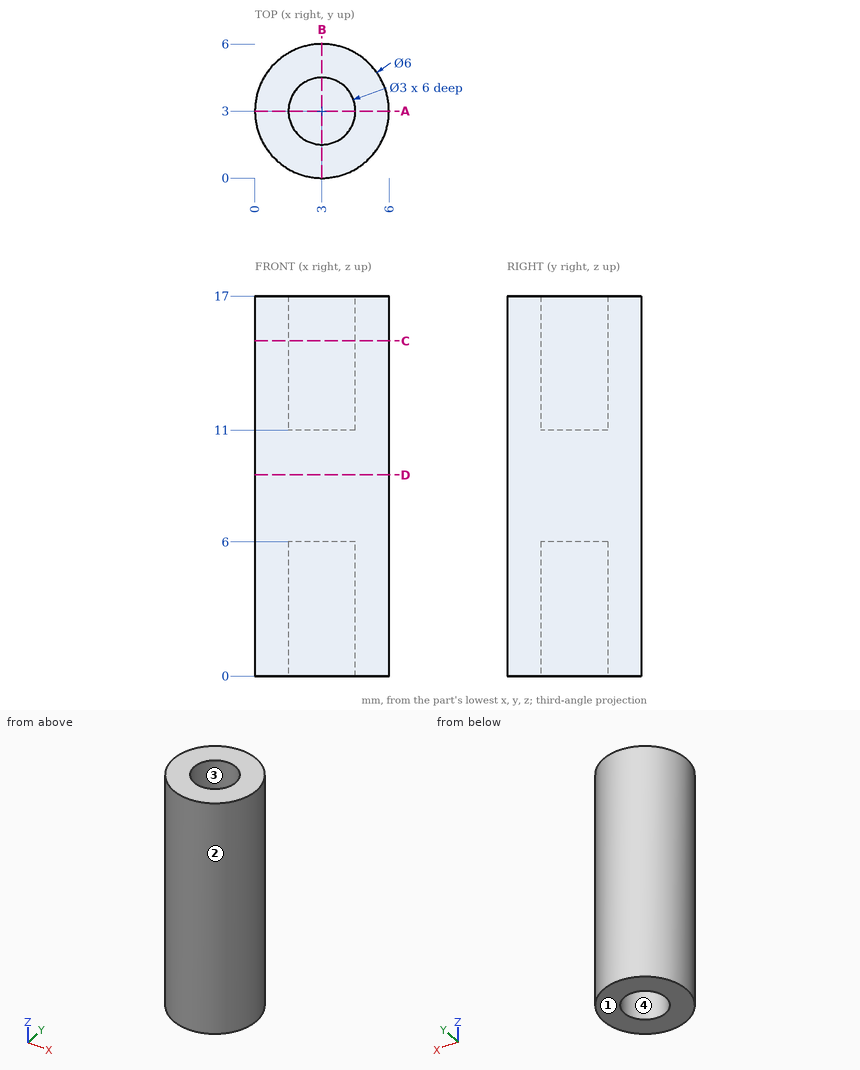
Answer from the drawing. Dimensions are ordinates in mm from the lowest x, y and z of the part. Give positions to 0.01 mm unless a question says otherwise; leave off trailing zeros. Loops run counter-clockwise (first coordinate to the right, second up) from the corner with the lowest first, then second, coordinate; pieces in that order, holes last. Notation, with made-up numbers: (74.5, -2.75) -> (83.5, -2.75) arc R24 cw to (83.5, 16.25) -> close; hole circle Ø4 at (63.5, -5). An arc over 180 degrees is marked (long way). Answer as CSV lines item,"result".
Item 1: Find section A-A on y = 3. Give the vertices of the cut face in (x, z).
Returned:
outline,"(0, 0) -> (1.5, 0) -> (1.5, 6) -> (4.5, 6) -> (4.5, 0) -> (6, 0) -> (6, 17) -> (4.5, 17) -> (4.5, 11) -> (1.5, 11) -> (1.5, 17) -> (0, 17) -> close"
Item 2: Find section C-C on z = 15. Give the vertices of the cut face in (x, y), plus the area to 3 significant figures.
Returned:
outline,"circle Ø6 at (3, 3); hole circle Ø3 at (3, 3)"
area,"21.2 mm²"
Item 3: Each of these flat-tipped pins is pushed along its axis until it touches: pin 1 (1 mm diameter, centred on x = 4, z = 14, fed in from -Y); pin 2 (0.9 mm diameter, centred on x = 3, y = 3.5, fed in from +Z); pin 3 (2 mm diameter, centred on y = 5, z = 12, fed in from +X). Where does it stop, or does it pass through?
Returned:
pin 1,"stops at y = 0.04"
pin 2,"stops at z = 11"
pin 3,"stops at x = 5.83"
Item 4: Consider line 1 (Y direction, x = 3, z = 1.6); line 2 (X direction, y = 3.7, z = 3.5). Determine where each line is inside the solid, lowest interval first. Write a range as [from, to].
Returned:
line 1,"y = [0, 1.5], [4.5, 6]"
line 2,"x = [0.08, 1.67], [4.33, 5.92]"
Item 5: Determine the mould class of the marked faces 1, 2, 3 and 4 for opening direction X: +X half, -X half, draft (parallel to the pull), parting line (faces both ways), or undercut.
Returned:
face 1,"draft"
face 2,"parting line"
face 3,"undercut"
face 4,"undercut"
Item 6: Find section D-D on z = 9. Give the vertices of the cut face in (x, y).
Returned:
outline,"circle Ø6 at (3, 3)"
